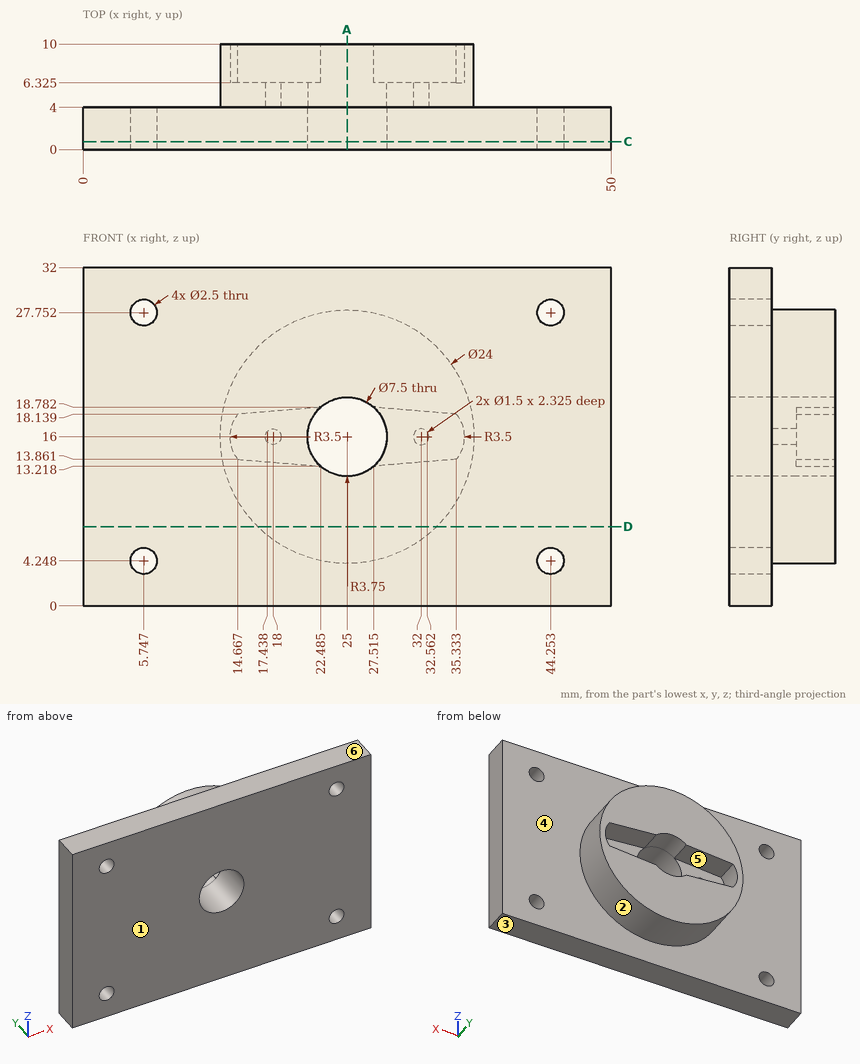
Design review of the part shown in the three views and the two pictorial views. Dimensions are in mm from the part's minimum x, y and z. A direction names the side the tool comes from. Give positions to 0.01 mm unless a question says otherwise; leave off trailing zeros. Loops run counter-clockwise (first coordinate to the right, second up) from the corner with the lowest first, then second, coordinate; pieces in that order, holes last. Notation, with made-up numbers: (5, -27) -> (35, -27) arc R17 cw to (35, -19) -> close; hole circle Ø7 at (-34.5, 43.25). An arc over 180 degrees is marked (long way). Write each question's results on one line, items separated by ' | '.
Q1. Take a section at A-A, the plane x = 25. Write out the cut boundary in (y, z), plus the area to 3 significant figures.
Reply:
outline: (0, 0) -> (4, 0) -> (4, 4) -> (10, 4) -> (10, 12.25) -> (0, 12.25) -> close; (0, 19.75) -> (10, 19.75) -> (10, 28) -> (4, 28) -> (4, 32) -> (0, 32) -> close | area: 197 mm²
Q2. Take a section at C-C, the plane y = 0.75. Write out the cut boundary in (x, z).
Reply:
outline: (0, 0) -> (50, 0) -> (50, 32) -> (0, 32) -> close; hole circle Ø2.5 at (5.75, 4.25); hole circle Ø2.5 at (5.75, 27.75); hole circle Ø7.5 at (25, 16); hole circle Ø2.5 at (44.25, 4.25); hole circle Ø2.5 at (44.25, 27.75)
Q3. For pin 1 Ø1.2 at (x, z) = (18, 16) entering from +Y; pin 2 Ø1.2 at (x, z) = (32, 15.5) entering from +Y (1 decimal); pin 3 Ø2 at (x, z) = (44.253, 4.248) entering from +Y, all flat-tipped, find the tip position at first contact; note any pin that passes through.
Reply:
pin 1: stops at y = 4 | pin 2: stops at y = 6.3 | pin 3: passes through
Q4. Take a section at D-D, the plane z = 7.5. Write out the cut boundary in (x, y), plus the area to 3 significant figures.
Reply:
outline: (0, 0) -> (50, 0) -> (50, 4) -> (33.47, 4) -> (33.47, 10) -> (16.53, 10) -> (16.53, 4) -> (0, 4) -> close | area: 302 mm²
Q5. Machinability: for the marked faces 1 and 2, which of the approach directions +Z, -Z, +X, -X, +Y, -Y give a long, thin tool a straight path to every point of the face, cutting with its end or side? Answer none if there is none.
Reply:
face 1: +Z, -Z, +X, -X, -Y | face 2: +Y
Q6. The part is to be moulded in two halves that separate along Z. For the marked faces 3, 4, 5 and 6, say which applies: +Z half, -Z half, draft (parallel to the pull), parting line (faces both ways), or undercut.
Reply:
face 3: -Z half | face 4: draft | face 5: undercut | face 6: +Z half
Q7. Wall thickness on L1, parallel to X at y = 4.5, z = 16; L2, parallel to X at y = 3.5, z = 16; L3, parallel to Y at x = 39, z = 28: over which ranges is each line inside the solid? List them lowest first.
Reply:
L1: x = 13 to 17.25, 18.75 to 21.25, 28.75 to 31.25, 32.75 to 37 | L2: x = 0 to 21.25, 28.75 to 50 | L3: y = 0 to 4
